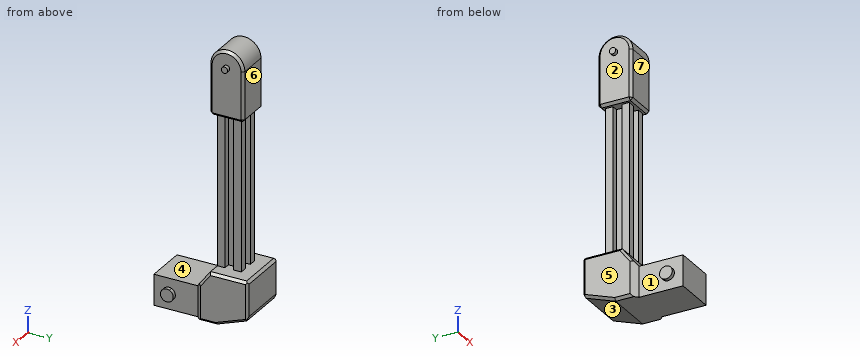
from build123d import *
from OCP.BRepFilletAPI import BRepFilletAPI_MakeChamfer

# Parameters (mm, degrees)
SKETCH_1_W          = 200
SKETCH_1_H          = 19
EXTRUDE_1_DEPTH     = 19
SKETCH_6_W          = 27
SKETCH_6_H          = 27
EXTRUDE_6_DEPTH     = 40
EXTRUDE_7_DEPTH     = 27
SKETCH_8_W          = 42.5
SKETCH_8_H          = 42.5
EXTRUDE_8_DEPTH     = 40
SKETCH_9_R          = 2.5
EXTRUDE_9_DEPTH     = 3
EXTRUDE_START       = 3
SKETCH_10_R         = 2.5
EXTRUDE_10_DEPTH    = 3
SKETCH_11_W         = 33
SKETCH_11_H         = 24.461700173
EXTRUDE_11_DEPTH    = 35
CUT_EXTRUDE_1_REACH = 211.742
CUT_EXTRUDE_2_DEPTH = 42.5
CUT_EXTRUDE_3_REACH = 222.711
SKETCH_15_W         = 120
SKETCH_15_H         = 7
CUT_EXTRUDE_4_DEPTH = 5
SKETCH_16_W         = 120
SKETCH_16_H         = 7
CUT_EXTRUDE_5_DEPTH = 5
SKETCH_17_W         = 7
SKETCH_17_H         = 120
CUT_EXTRUDE_6_DEPTH = 5
SKETCH_18_W         = 7
SKETCH_18_H         = 120
CUT_EXTRUDE_7_DEPTH = 5
CHAMFER_1_SIZE      = 2
CHAMFER_2_SIZE      = 2
CHAMFER_3_SIZE      = 2
CHAMFER_3_SIZE2     = 3.330930275
CHAMFER_4_SIZE      = 2
BOSS_EXTRUDE1_DEPTH = 3
BOSS_EXTRUDE2_START = 3
BOSS_EXTRUDE2_DEPTH = 3


with BuildPart() as part:
    # 草图1 → 凸台-拉伸1 (new body)
    with BuildSketch(Plane(origin=(0, 0, 0), x_dir=(0, 0, -1), z_dir=(1, 0, 0))):
        with Locations((100, 9.5)):
            Rectangle(SKETCH_1_W, SKETCH_1_H)
    extrude(amount=EXTRUDE_1_DEPTH)

    # 草图6 → 凸台-拉伸6 (add)
    with BuildSketch(Plane.XY):
        with Locations((9.5, 9.5)):
            Rectangle(SKETCH_6_W, SKETCH_6_H)
    extrude(amount=-EXTRUDE_6_DEPTH)

    # 草图7 → 凸台-拉伸7 (add)
    with BuildSketch(Plane(origin=(23, 0, 0), x_dir=(0, 0, -1), z_dir=(1, 0, 0))):
        with BuildLine():
            Line((0, -4), (0, 23))
            ThreePointArc((0, 23), (-13.5, 9.5), (0, -4))
        make_face()
    extrude(amount=-EXTRUDE_7_DEPTH)

    # 草图8 → 凸台-拉伸8 (add)
    with BuildSketch(Plane(origin=(0, 0, -200), x_dir=(-1, 0, 0), z_dir=(0, 0, -1))):
        with Locations((-9.5, 9.5)):
            Rectangle(SKETCH_8_W, SKETCH_8_H)
    extrude(amount=-EXTRUDE_8_DEPTH)

    # 草图9 → 凸台-拉伸9 (add)
    with BuildSketch(Plane(origin=(23, 0, 0), x_dir=(0, 0, -1), z_dir=(1, 0, 0))):
        with Locations((0, 9.5)):
            Circle(SKETCH_9_R)
    extrude(amount=EXTRUDE_9_DEPTH)

    # 草图10 → 凸台-拉伸10 (add)
    with BuildSketch(Plane.ZY.offset(4).offset(EXTRUDE_START)):
        with Locations(Location((0, 9.5, 0), (0, 0, 180))):
            Circle(SKETCH_10_R)
    extrude(amount=-EXTRUDE_10_DEPTH)

    # 草图11 → 凸台-拉伸11 (add)
    with BuildSketch(Plane.XZ.offset(11.75)):
        with Locations((9.5, -187.769149914)):
            Rectangle(SKETCH_11_W, SKETCH_11_H)
    extrude(amount=EXTRUDE_11_DEPTH)

    # 切除-拉伸1: up to this face of the body (flat: up to its plane)
    cut_extrude_1_end = Plane(part.part.faces().sort_by_distance((-11.75, 9.5, -180))[0])
    # 草图12 → 切除-拉伸1 (cut, up to the picked face)
    with BuildSketch(Plane(origin=(30.75, 0, 0), x_dir=(0, 0, -1), z_dir=(1, 0, 0)), mode=Mode.PRIVATE) as cut_extrude_1_sk1:
        Polygon((160, 0), (175.538299827, -11.75), (160, -11.75), align=None)
    cut_extrude_1_tool1 = split(extrude(cut_extrude_1_sk1.sketch, amount=-CUT_EXTRUDE_1_REACH, mode=Mode.PRIVATE), bisect_by=cut_extrude_1_end, keep=Keep.BOTH, mode=Mode.PRIVATE)
    add(cut_extrude_1_tool1.solids().sort_by(Axis((30.75, -7.833333, -165.179433), (-1, 0, 0)))[0], mode=Mode.SUBTRACT)

    # 草图13 → 切除-拉伸2 (cut)
    with BuildSketch(Plane.ZY.offset(11.75)):
        Polygon((-190.839141878, 30.75), (-200, 5.410999189), (-200, 30.75), align=None)
    extrude(amount=-CUT_EXTRUDE_2_DEPTH, mode=Mode.SUBTRACT)

    # 切除-拉伸3: up to this plane
    cut_extrude_3_end = Plane(origin=(-31.230792117, 0, -160), z_dir=(0, 0.7976215614630531, -0.603158225252082))
    # 草图14 → 切除-拉伸3 (cut, up to the surface)
    with BuildSketch(Plane(origin=(0, 0, -200), x_dir=(-1, 0, 0), z_dir=(0, 0, -1)), mode=Mode.PRIVATE) as cut_extrude_3_sk1:
        Polygon((-26, -11.75), (-30.75, -7), (-30.75, -11.75), align=None)
    cut_extrude_3_tool1 = split(extrude(cut_extrude_3_sk1.sketch, amount=-CUT_EXTRUDE_3_REACH, mode=Mode.PRIVATE), bisect_by=cut_extrude_3_end, keep=Keep.BOTH, mode=Mode.PRIVATE)
    add(cut_extrude_3_tool1.solids().sort_by_distance((29.166667, -10.166667, -200))[0], mode=Mode.SUBTRACT)
    # 草图14 → 切除-拉伸3 (cut, up to the surface)
    with BuildSketch(Plane(origin=(0, 0, -200), x_dir=(-1, 0, 0), z_dir=(0, 0, -1)), mode=Mode.PRIVATE) as cut_extrude_3_sk2:
        Polygon((7, -11.75), (11.75, -7), (11.75, -11.75), align=None)
    cut_extrude_3_tool2 = split(extrude(cut_extrude_3_sk2.sketch, amount=-CUT_EXTRUDE_3_REACH, mode=Mode.PRIVATE), bisect_by=cut_extrude_3_end, keep=Keep.BOTH, mode=Mode.PRIVATE)
    add(cut_extrude_3_tool2.solids().sort_by_distance((-10.166667, -10.166667, -200))[0], mode=Mode.SUBTRACT)

    # 草图15 → 切除-拉伸4 (cut)
    with BuildSketch(Plane.ZY):
        with Locations((-100, 9.5)):
            Rectangle(SKETCH_15_W, SKETCH_15_H)
    extrude(amount=-CUT_EXTRUDE_4_DEPTH, mode=Mode.SUBTRACT)

    # 草图16 → 切除-拉伸5 (cut)
    with BuildSketch(Plane(origin=(19, 0, 0), x_dir=(0, 0, -1), z_dir=(1, 0, 0))):
        with Locations((100, 9.5)):
            Rectangle(SKETCH_16_W, SKETCH_16_H)
    extrude(amount=-CUT_EXTRUDE_5_DEPTH, mode=Mode.SUBTRACT)

    # 草图17 → 切除-拉伸6 (cut)
    with BuildSketch(Plane.XZ):
        with Locations((9.5, -100)):
            Rectangle(SKETCH_17_W, SKETCH_17_H)
    extrude(amount=-CUT_EXTRUDE_6_DEPTH, mode=Mode.SUBTRACT)

    # 草图18 → 切除-拉伸7 (cut)
    with BuildSketch(Plane(origin=(0, 19, 0), x_dir=(1, 0, 0), z_dir=(0, 1, 0))):
        with Locations((9.5, 100)):
            Rectangle(SKETCH_18_W, SKETCH_18_H)
    extrude(amount=-CUT_EXTRUDE_7_DEPTH, mode=Mode.SUBTRACT)

    # 倒角1
    chamfer_1_edges = [part.edges().sort_by_distance(p)[0] for p in [
        (30.75, 18.080499595, -195.419570939),
        (30.75, -3.5, -164.628429736),
        (30.75, 15.375, -160),
        (30.75, 30.75, -175.419570939),
        (30.75, -0.794500405, -200),
    ]]
    chamfer(chamfer_1_edges, length=CHAMFER_1_SIZE)

    # 倒角2
    chamfer_2_edges = [part.edges().sort_by_distance(p)[0] for p in [
        (-11.75, -3.5, -164.628429736),
        (-11.75, -0.794500405, -200),
        (-11.75, 30.75, -175.419570939),
        (-11.75, 15.375, -160),
        (-11.75, 18.080499595, -195.419570939),
    ]]
    chamfer(chamfer_2_edges, length=CHAMFER_2_SIZE)

    # 倒角3: one chamfer whose edges measure the first distance from different faces: ONE call of the kernel's chamfer builder (chamfer() names one face for all edges)
    chamfer_3_edges_1 = [part.edges().sort_by_distance(p)[0] for p in [
        (9.5, 30.75, -190.839141878),
    ]]
    chamfer_3_side_1 = [part.faces().sort_by_distance(p)[0] for p in [
        (9.5, 18.080499595, -195.419570939),
    ]]
    chamfer_3_edges_2 = [part.edges().sort_by_distance(p)[0] for p in [
        (9.5, 30.75, -160),
    ]]
    chamfer_3 = BRepFilletAPI_MakeChamfer(part.part.solid().wrapped)
    for e in chamfer_3_edges_1:
        chamfer_3.Add(CHAMFER_3_SIZE, CHAMFER_3_SIZE2, e.wrapped, chamfer_3_side_1[0].wrapped)  # the first distance lies on this face
    for e in chamfer_3_edges_2:
        chamfer_3.Add(CHAMFER_3_SIZE, e.wrapped)
    add(Compound.cast(chamfer_3.Shape()), mode=Mode.REPLACE)

    # 倒角4
    chamfer_4_edges = [part.edges().sort_by_distance(p)[0] for p in [
        (23, 9.5, -40),
        (23, 23, -20),
        (9.5, -4, -40),
        (23, -4, -20),
        (-4, 9.5, -40),
        (-4, -4, -20),
        (9.5, 23, -40),
        (-4, 23, -20),
        (23, 9.5, 13.5),
        (-4, 9.5, 13.5),
    ]]
    chamfer(chamfer_4_edges, length=CHAMFER_4_SIZE)

    # Sketch2 → Boss-Extrude1 (add)
    with BuildSketch(Plane.ZY.offset(7)):
        with BuildLine():
            ThreePointArc((-182.669149914, -34.75), (-182.770150014, -33.740049506), (-183.069149914, -32.770101013))
            ThreePointArc((-183.069149914, -32.770101013), (-187.769149914, -29.65), (-192.469149914, -32.770101013))
            ThreePointArc((-192.469149914, -32.770101013), (-188.779100407, -39.7489999), (-182.669149914, -34.75))
        make_face()
    extrude(amount=BOSS_EXTRUDE1_DEPTH)

    # Sketch3 → Boss-Extrude2 (add)
    with BuildSketch(Plane(origin=(26, 0, 0), x_dir=(0, 0, -1), z_dir=(1, 0, 0)).offset(BOSS_EXTRUDE2_START)):
        with BuildLine():
            ThreePointArc((192.869149914, -34.75), (192.768149814, -33.740049506), (192.469149914, -32.770101013))
            ThreePointArc((192.469149914, -32.770101013), (187.769149914, -29.65), (183.069149914, -32.770101013))
            ThreePointArc((183.069149914, -32.770101013), (186.75919942, -39.7489999), (192.869149914, -34.75))
        make_face()
    extrude(amount=-BOSS_EXTRUDE2_DEPTH)


solid = part.part
The listing builds one solid part. Answer for the finished solid, in the listing's coordinates (mm). Face numbers are marked on the shaded views. A direction names the side the tool comes from. Coordinates: 2 decimals unless noted, no trailing zeros. Order: outer loops, then holes, each group sorted by start corner. A loop starts at its lowest first (then second) coordinate and runs counter-clockwise, first axis right, second up.
Q1. Which of the six approach directions +Z, -Z, +X, -X, +Y, -Y give full straight-line access (tool end or side, diameter ignored) to the marked faces 5, 6 and 7?
Q2. For a pull along Z with two mould halves and no side action, classify the marked faces 1, 2, 3 and 4 as pulls with the +Z half, pulls with the -Z half, needs draft (parallel to the pull), parting line crosses it, or undercut.
Q3. A cutting plane is placed at C-C, the plane z = -42.5. Write down the section's boundary in (x, y).
Q4. Given P1, Ø2, axis at x = 16.5, y = 13.5, coming from the -Z side; P2, Ø5, axis at y = 4, z = -75.5, coming from the +X side; P3, Ø4, axis at x = 1.5, z = -79, coming from the +Y side, each flat-ended and moving along its own axis, determine where each tip first touches the part or whether it passes through.
Q5. A cutting plane is placed at B-B, the plane y = 9.5. Write down the section's boundary in (x, z) (3 decimals), and give its area (3 significant figures).
Q6. A cutting plane is placed at D-D, the plane y = -27. Write down the section's boundary in (x, z).
Q7. Consider line 1 (Y direction, x = 3, z = -85); line 2 (X direction, y = 9, z = -124.5). Determine where each line is inside the solid, lowest interval first.
Q8. A cutting plane is placed at A-A, the plane z = -19.5. Write down the section's boundary in (x, y).
Answers follow:
1. face 5: +Z, -Z, -X, +Y, -Y
1. face 6: +Z, +X, -X, +Y
1. face 7: +Z, +X, -X, -Y
2. face 1: needs draft
2. face 2: undercut
2. face 3: pulls with the -Z half
2. face 4: pulls with the +Z half
3. outline: (0, 0) - (6, 0) - (6, 5) - (13, 5) - (13, 0) - (19, 0) - (19, 6) - (14, 6) - (14, 13) - (19, 13) - (19, 19) - (13, 19) - (13, 14) - (6, 14) - (6, 19) - (0, 19) - (0, 13) - (5, 13) - (5, 6) - (0, 6) - close
4. P1: stops at z = -197.44
4. P2: stops at x = 19
4. P3: stops at y = 19
5. outline: (-11.75, -196.395) - (-9.75, -198.522) - (28.75, -198.522) - (30.75, -196.395) - (30.75, -162) - (28.75, -160) - (14, -160) - (14, -40) - (21, -40) - (23, -38) - (23, -2.5) - (26, -2.5) - (26, 2.5) - (23, 2.5) - (23, 11.5) - (21, 13.5) - (-2, 13.5) - (-4, 11.5) - (-4, 2.5) - (-7, 2.5) - (-7, -2.5) - (-4, -2.5) - (-4, -38) - (-2, -40) - (5, -40) - (5, -160) - (-9.75, -160) - (-11.75, -162) - close
5. area: 4,180 mm2
6. outline: (-7, -200) - (26, -200) - (26, -175.54) - (-7, -175.54) - close
7. line 1: y = 0 to 6, 13 to 19
7. line 2: x = 5 to 14
8. outline: (-4, -2) - (-2, -4) - (21, -4) - (23, -2) - (23, 21) - (21, 23) - (-2, 23) - (-4, 21) - close
